Autodesk Fusion 360 part; units mm, degrees
sketch "Sketch1" plane through (0, 0, 0) normal (0, 0, 1) x (1, 0, 0)
  circle A0 centre (0, 0) radius 25
  line L0 (10, -45) -> (-10, -45)
  line L1 (-10, -45) -> (-10, 45)
  line L2 (-10, 45) -> (10, 45)
  line L3 (10, 45) -> (10, -45)
  line L4 (10, -45) -> (-10, 45) construction
  line L5 (-10, -45) -> (10, 45) construction
  dimension "d1" = 50
  dimension "d2" = 90
  dimension "d3" = 20
extrude "Extrude1" add sketch "Sketch1" against normal blind 1.5 contours A0 L3 | A0 L1 L3 | A0 L0 L1 L3 | A0 L1
fillet "Fillet1" radius 8 2 edges at (-10, -45, -0.75) (10, -45, -0.75)
fillet "Fillet2" radius 5 2 edges at (-10, -22.9129, -0.75) (10, -22.9129, -0.75)
sketch "Sketch2" plane through (0, 0, 0) normal (0, 0, 1) x (-1, 0, 0)
  line L0 (-10, 37) -> (-10, 25.9808)
  arc A0 (-12.5, 21.6506) -> (12.5, 21.6506) centre (0, 0) ccw
  line L1 (10, 25.9808) -> (10, 37)
  line L2 (2, 45) -> (-2, 45)
  line L3 (-10, 33) -> (-3, 33)
  line L4 (-0.5, 28.9564) -> (-0.5, 37.0436)
  arc A1 (-0.5, 37.0436) -> (-5.5, 37.0436) centre (-3, 37.0436) ccw
  line L5 (-5.5, 37.0436) -> (-5.5, 28.9564)
  arc A2 (-5.5, 28.9564) -> (-0.5, 28.9564) centre (-3, 28.9564) ccw
  line L6 (-3, 28.9564) -> (-3, 37.0436) construction
  line L7 (1.7, 28.9564) -> (1.7, 37.0436)
  arc A3 (1.7, 37.0436) -> (-7.7, 37.0436) centre (-3, 37.0436) ccw
  line L8 (-7.7, 37.0436) -> (-7.7, 28.9564)
  arc A4 (-7.7, 28.9564) -> (1.7, 28.9564) centre (-3, 28.9564) ccw
  arc A5 (-2, 45) -> (-10, 37) centre (-2, 37) ccw
  arc A6 (-12.5, 21.6506) -> (-10, 25.9808) centre (-15, 25.9808) ccw
  arc A7 (10, 25.9808) -> (12.5, 21.6506) centre (15, 25.9808) ccw
  arc A8 (10, 37) -> (2, 45) centre (2, 37) ccw
  line L9 (-9, 37) -> (-9, 25.9808)
  arc A9 (-12, 20.7846) -> (-9, 25.9808) centre (-15, 25.9808) ccw
  arc A10 (-12, 20.7846) -> (12, 20.7846) centre (0, 0) ccw
  arc A11 (9, 25.9808) -> (12, 20.7846) centre (15, 25.9808) ccw
  line L10 (9, 25.9808) -> (9, 37)
  arc A12 (9, 37) -> (2, 44) centre (2, 37) ccw
  line L11 (2, 44) -> (-2, 44)
  arc A13 (-2, 44) -> (-9, 37) centre (-2, 37) ccw
  point P0 (-3, 33)
  dimension "d6" = 7
  dimension "d7" = 5
  dimension "d8" = 2.2
  dimension "d14" = 1
extrude "Extrude2" add sketch "Sketch2" along normal blind 0.2 contours L4 A1 L5 A2 | L9 A9 A10 A11 L10 A12 L11 A13
Read the model definition and answer for the solid it produces. Units are mm, in the model's axes. A direction names the side the tool comes from. Give positions to 0.01 mm unless a question says otherwise; leave off trailing zeros. Order: outer loops, then holes, each group sorted by start corner. A loop starts at its lowest first (then second) coordinate and runs counter-clockwise, first axis right, second up. Notation, with made-up numbers: (82.5, -19.5) -> (139.5, -19.5) arc R33 cw to (139.5, 10.5) -> close; hole circle Ø3 at (-16, 40.25). An arc over 180 degrees is marked (long way). Write item = value, one per line.
1. A cutting plane is placed at A-A, the plane z = -0.85. Write down the section's boundary in (x, y).
Numbers:
outline = (-12.5, -21.65) arc R5 cw to (-10, -25.98) -> (-10, -37) arc R8 ccw to (-2, -45) -> (2, -45) arc R8 ccw to (10, -37) -> (10, -25.98) arc R5 cw to (12.5, -21.65) arc R25 ccw (long way) to start
2. A cutting plane is placed at B-B, the plane y = -30. Write down the section's boundary in (x, z), and give its area (3 significant figures).
Numbers:
outline = (-10, -1.5) -> (10, -1.5) -> (10, 0) -> (9, 0) -> (9, 0.2) -> (7.7, 0.2) -> (7.7, 0) -> (5.5, 0) -> (5.5, 0.2) -> (0.5, 0.2) -> (0.5, 0) -> (-1.7, 0) -> (-1.7, 0.2) -> (-9, 0.2) -> (-9, 0) -> (-10, 0) -> close
area = 32.7 mm²
3. The mould has two halves that part along Y. Classify faces 1 (the face through (0.916, 24.983, -0.74)), 2 (the face through (-7.594, -42.719, -0.76)), 3 (the face through (6, -33, 0)), 4 (the face through (0, -3, 0.2)): +Y half, -Y half, draft (parallel to the pull), parting line (faces both ways), or undercut.
Numbers:
face_1 = parting line
face_2 = -Y half
face_3 = undercut
face_4 = draft
4. Straight lines are drawn through the part: line 1 along Z through (x, y) = (1, -25); line 2 along X through (y, z) = (7, -0.05); line 3 along X through (y, z) = (-37, -0.05). For each, find the intervals that lie inside material, in ascending order.
Numbers:
line_1 = -1.5 to 0
line_2 = -24 to 24
line_3 = -10 to 10
5. A cutting plane is placed at C-C, the plane x = -16. Write down the section's boundary in (y, z).
Numbers:
outline = (-19.21, -1.5) -> (19.21, -1.5) -> (19.21, 0) -> (17.89, 0) -> (17.89, 0.2) -> (-17.89, 0.2) -> (-17.89, 0) -> (-19.21, 0) -> close
6. For faces 5 (the face through (-10, -32, -1)), 6 (the face through (10.652, -23.513, -0.76)), determine the directions among +Z, -Z, +X, -X, +Y, -Y from which every point of the face is accessible in a straight line to the end or side of a thin tool.
Numbers:
face_5 = +Z, -Z, -X, -Y
face_6 = +Z, -Z, +X, -Y
